Can you work these out from the model? Positions are in its coordinate system, mm. Face numbers are marked on the shaded views. A direction names the side the tool comes from. Round coordinates to 2 decimals unless told otherwise and drop trailing zeros. Loops run counter-clockwise (first coordinate to the right, second up) from the corner with the lowest first, then second, coordinate; pieces in that order, holes last.
(1) Will these pins go through, and if not, where does the flat tip stop? pin 1 Ø6 at (x, y) = (27.5, -31.5) entering from -Z; pin 2 Ø7.5 at (x, z) = (63, -7) entering from +Y.
(2) I want a section at B-B on x = 50. Write out the boundary of the cut face in (y, z).
(3) Which directions (+Z, -Z, +X, -X, +Y, -Y) give clear straight access to the entire face, cutting with the end or side of a thin tool? Please do the marked faces 1 and 2.
(4) Thinking about a two-plate mould opening in Y: for the marked faces 3, 4 and 5, which applies, released by +Y, released by -Y, zero draft, split by the parting line, or undercut?
(5) If I drill on line 1 along Z through (x, y) = (17.5, -39); line 2 along X through (y, z) = (36.5, 3.5); line 3 along Y through (x, z) = (96, -4), over which ranges is the centre line in solid material (lowest first)?
(6) I want a section at A-A on x = 82.5. Write out the boundary of the cut face in (y, z).
(7) I want a section at D-D on y = -38.5. Write out the boundary of the cut face in (x, z).
(8) I want a section at C-C on z = -8.5. Write out the boundary of the cut face in (x, y).
from build123d import *

# Parameters (mm, degrees)
EXTRUDE_1_DEPTH     = 10
SKETCH_2_W          = 169.882057187
SKETCH_2_H          = 25.097327733
CUT_EXTRUDE_1_DEPTH = 11
SKETCH_4_W          = 150
SKETCH_4_H          = 103
EXTRUDE_2_DEPTH     = 10
SKETCH_5_W          = 50
SKETCH_5_H          = 103
CUT_EXTRUDE_2_DEPTH = 11
SKETCH_7_W          = 130.949422717
SKETCH_7_H          = 60
CUT_EXTRUDE_3_DEPTH = 10
SKETCH_8_R          = 5
CUT_EXTRUDE_4_DEPTH = 11
CUT_EXTRUDE_5_DEPTH = 11
SKETCH_12_W         = 100
SKETCH_12_H         = 10
EXTRUDE_3_DEPTH     = 45
SKETCH_13_W         = 100
SKETCH_13_H         = 5
EXTRUDE_4_DEPTH     = 25
SKETCH_14_W         = 100
SKETCH_14_H         = 15
EXTRUDE_5_DEPTH     = 5
SKETCH_15_R         = 2.75
CUT_EXTRUDE_6_DEPTH = 11


with BuildPart() as part:
    # 草图1 → 凸台-拉伸1 (new body)
    with BuildSketch(Plane.XY):
        Polygon((150, 103.55), (0, 90.426700471), (0, 0), (150, 0), align=None)
    extrude(amount=EXTRUDE_1_DEPTH)

    # 草图2 → 切除-拉伸1 (cut, through all)
    with BuildSketch(Plane(origin=(0, 0, 0), x_dir=(-1, 0, 0), z_dir=(0, 0, -1))):
        with Locations((-84.941028594, 102.975364337)):
            Rectangle(SKETCH_2_W, SKETCH_2_H)
    extrude(amount=-CUT_EXTRUDE_1_DEPTH, mode=Mode.SUBTRACT)

    # 草图4 → 凸台-拉伸2 (add)
    with BuildSketch(Plane.XY.offset(10)):
        with Locations((75, 51.5)):
            Rectangle(SKETCH_4_W, SKETCH_4_H)
    extrude(amount=-EXTRUDE_2_DEPTH)

    # 草图5 → 切除-拉伸2 (cut, through all)
    with BuildSketch(Plane.XY.offset(10)):
        with Locations((125, 51.5)):
            Rectangle(SKETCH_5_W, SKETCH_5_H)
    extrude(amount=-CUT_EXTRUDE_2_DEPTH, mode=Mode.SUBTRACT)

    # 草图7 → 切除-拉伸3 (cut)
    with BuildSketch(Plane.XY.offset(10)):
        with Locations((65.474711359, 73)):
            Rectangle(SKETCH_7_W, SKETCH_7_H)
    extrude(amount=-CUT_EXTRUDE_3_DEPTH, mode=Mode.SUBTRACT)

    # 草图8 → 切除-拉伸4 (cut, through all)
    with BuildSketch(Plane(origin=(0, 0, 0), x_dir=(-1, 0, 0), z_dir=(0, 0, -1))):
        with Locations((-50, 33)):
            Circle(SKETCH_8_R)
    extrude(amount=-CUT_EXTRUDE_4_DEPTH, mode=Mode.SUBTRACT)

    # 草图11 → 切除-拉伸5 (cut, through all)
    with BuildSketch(Plane(origin=(0, 0, 0), x_dir=(-1, 0, 0), z_dir=(0, 0, -1))):
        with BuildLine():
            ThreePointArc((-76.764545578, 23.96), (-72.645438565, 21.920892987), (-70.606331551, 26.04))
            ThreePointArc((-70.606331551, 26.04), (-71.707959146, 31.648330774), (-71.310560762, 37.35))
            ThreePointArc((-71.310560762, 37.35), (-73.844897428, 41.184336666), (-77.679234093, 38.65))
            ThreePointArc((-77.679234093, 38.65), (-78.195395213, 31.24438365), (-76.764545578, 23.96))
        make_face()
    cut_extrude_5 = extrude(amount=-CUT_EXTRUDE_5_DEPTH, mode=Mode.SUBTRACT)

    # 镜向1: 切除-拉伸5 across plane
    add(cut_extrude_5.mirror(Plane.ZY.offset(-50)), mode=Mode.SUBTRACT)

    # 草图12 → 凸台-拉伸3 (add)
    with BuildSketch(Plane.XZ):
        with Locations((50, 5)):
            Rectangle(SKETCH_12_W, SKETCH_12_H)
    extrude(amount=EXTRUDE_3_DEPTH)

    # 草图13 → 凸台-拉伸4 (add)
    with BuildSketch(Plane.XY.offset(10)):
        with Locations((50, -42.5)):
            Rectangle(SKETCH_13_W, SKETCH_13_H)
    extrude(amount=-EXTRUDE_4_DEPTH)

    # 草图14 → 凸台-拉伸5 (add)
    with BuildSketch(Plane(origin=(0, -40, 0), x_dir=(1, 0, 0), z_dir=(0, 1, 0))):
        with Locations((50, 7.5)):
            Rectangle(SKETCH_14_W, SKETCH_14_H)
    extrude(amount=EXTRUDE_5_DEPTH)

    # 草图15 → 切除-拉伸6 (cut, through all)
    with BuildSketch(Plane(origin=(0, -35, 0), x_dir=(1, 0, 0), z_dir=(0, 1, 0))):
        with Locations((82.5, 6.885250494)):
            Circle(SKETCH_15_R)
        with Locations((17.5, 6.885250494)):
            Circle(SKETCH_15_R)
    extrude(amount=-CUT_EXTRUDE_6_DEPTH, mode=Mode.SUBTRACT)


solid = part.part
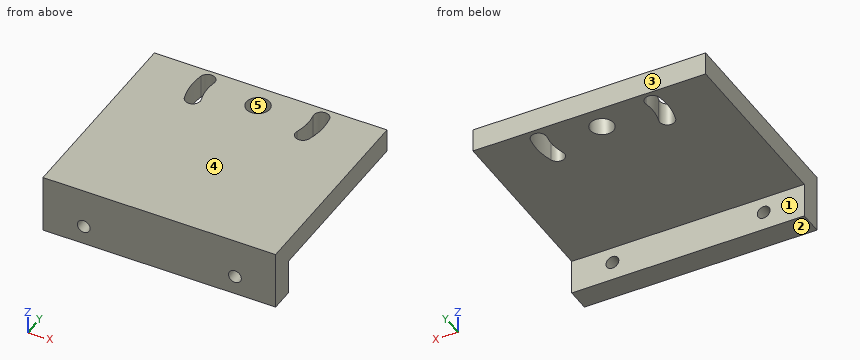
Filled sheet:
1. pin 1: stops at z = 0
1. pin 2: stops at y = -35
2. outline: (-45, -15) - (-35, -15) - (-35, 0) - (28, 0) - (28, 10) - (-45, 10) - close; (38, 0) - (43, 0) - (43, 10) - (38, 10) - close
3. face 1: -Z, +X, -X, +Y
3. face 2: -Z, +X, -X, +Y, -Y
4. face 3: released by +Y
4. face 4: zero draft
4. face 5: undercut
5. line 1: z = -15 to -9.64, -4.14 to 10
5. line 2: x = 0 to 21.97, 28.53 to 46.43, 53.57 to 71.47, 78.03 to 100
5. line 3: y = -45 to -35
6. outline: (-45, -15) - (-35, -15) - (-35, -9.64) - (-45, -9.64) - close; (-45, -4.14) - (-35, -4.14) - (-35, 0) - (43, 0) - (43, 10) - (-45, 10) - close
7. outline: (0, -15) - (100, -15) - (100, 10) - (0, 10) - close; hole circle Ø5.5 at (17.5, -6.89); hole circle Ø5.5 at (82.5, -6.89)
8. outline: (0, -45) - (15.27, -45) - (15.27, -35) - (0, -35) - close; (19.73, -45) - (80.27, -45) - (80.27, -35) - (19.73, -35) - close; (84.73, -45) - (100, -45) - (100, -35) - (84.73, -35) - close
